Answer from the drawing. Dimensions are ordinates in mm from the lowest x, y and z of the part. A direction names the side the tool comes from. Round coordinates to 2 decimals unless told otherwise and drop trailing zeros. Loops run counter-clockwise (first coordinate to the right, second up) from the corner with the lowest first, then second, coordinate; pieces in that order, holes last. Notation, with made-up numbers: (54.5, -0.75) -> (100.5, -0.75) arc R15 ccw to (100.5, 21.25) -> close; hole circle Ø11 at (63, 51.5). An arc over 180 degrees is marked (long way). One line per question, with ' | ' between items.
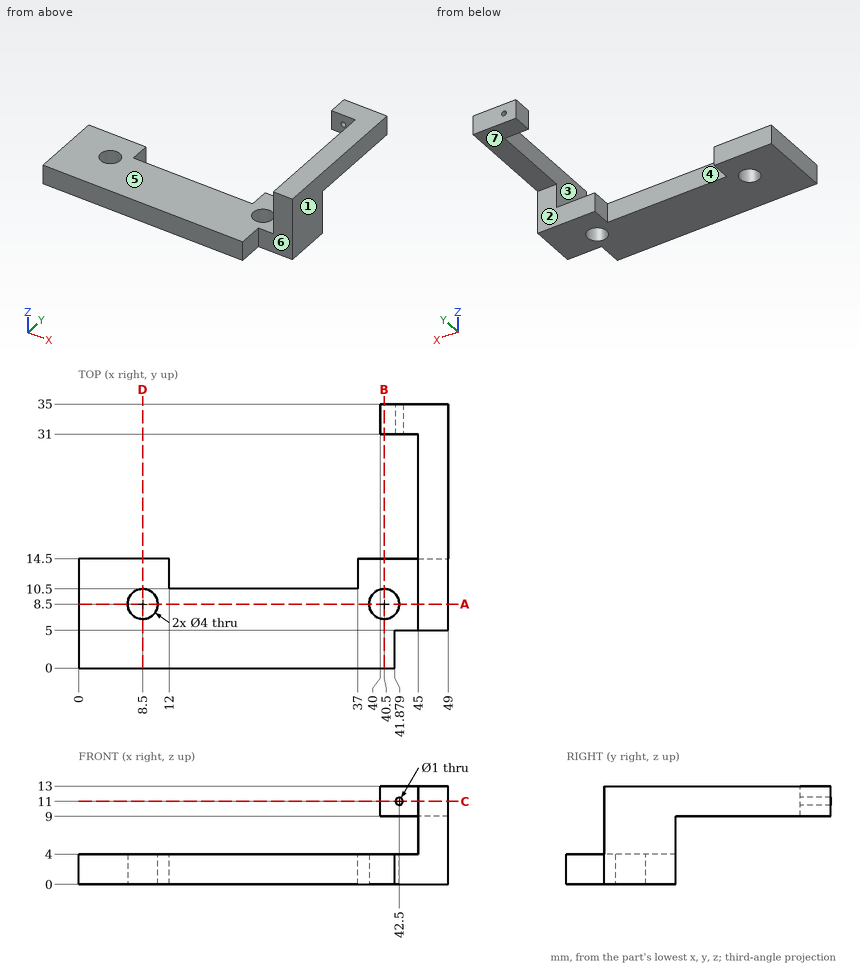
Q1. A cutting plane is placed at C-C on z = 11. Give the vertices of the cut face in (x, y).
Numbers:
outline: (40, 31) -> (42, 31) -> (42, 35) -> (40, 35) -> close; (43, 31) -> (45, 31) -> (45, 5) -> (49, 5) -> (49, 35) -> (43, 35) -> close
Q2. Given pin 1 Ø3 at (x, y) = (34.5, 11.5) entering from +Z; pin 2 Ø1.2 at (x, z) = (22, 2) entering from +Y; pin 3 Ø2 at (y, z) = (32.5, 11) entering from -X, each flat-ended and moving along its own axis, determine where each tip first touches the part or whether it passes through.
Numbers:
pin 1: z = 4 | pin 2: y = 10.5 | pin 3: x = 40
Q3. A cutting plane is placed at D-D on x = 8.5. Give the vertices of the cut face in (y, z), plus the area to 3 significant figures.
Numbers:
outline: (0, 0) -> (6.5, 0) -> (6.5, 4) -> (0, 4) -> close; (10.5, 0) -> (14.5, 0) -> (14.5, 4) -> (10.5, 4) -> close | area: 42.0 mm^2
Q4. Find the intervals of material crossed by line 1 (Y direction, x = 8.5, z = 2.6); line 2 (X direction, y = 8.5, z = 2.6); line 3 (Z direction, x = 42.5, y = 32.3), in increasing order. Write a range as from..to.
Numbers:
line 1: 0..6.5, 10.5..14.5 | line 2: 0..6.5, 10.5..38.5, 42.5..49 | line 3: 9..10.5, 11.5..13
Q5. For a pull along X with two mould halves and no side action, classify the marked faces 1, 2, 3 and 4 as pulls with the +X half, pulls with the -X half, needs draft (parallel to the pull), parting line crosses it, or undercut.
Numbers:
face 1: pulls with the +X half | face 2: needs draft | face 3: pulls with the -X half | face 4: undercut
Q6. A cutting plane is placed at A-A on y = 8.5. Give the vertices of the cut face in (x, z), plus the area to 3 significant figures.
Numbers:
outline: (0, 0) -> (6.5, 0) -> (6.5, 4) -> (0, 4) -> close; (10.5, 0) -> (38.5, 0) -> (38.5, 4) -> (10.5, 4) -> close; (42.5, 0) -> (49, 0) -> (49, 13) -> (45, 13) -> (45, 4) -> (42.5, 4) -> close | area: 200 mm^2
Q7. A cutting plane is placed at B-B on x = 40.5. Give the vertices of the cut face in (y, z), plus the area to 3 significant figures.
Numbers:
outline: (0, 0) -> (6.5, 0) -> (6.5, 4) -> (0, 4) -> close; (10.5, 0) -> (14.5, 0) -> (14.5, 4) -> (10.5, 4) -> close; (31, 9) -> (35, 9) -> (35, 13) -> (31, 13) -> close | area: 58.0 mm^2
Q8. For the marked faces 5, 6 and 7, determine the directions among +Z, -Z, +X, -X, +Y, -Y from which every point of the face is accessible in a straight line to the end or side of a thin tool.
Numbers:
face 5: +Z, -X, +Y, -Y | face 6: +Z, -Z, +X, -Y | face 7: -Z, +X, -X, +Y
